The listing builds one solid part. Answer for the finished solid, in the listing's coordinates (mm). Coordinates: 2 decimals unless noted, no trailing zeros. Order: outer loops, then holes, each group sorted by start corner. A loop starts at its lowest first (then second) coordinate and runs counter-clockwise, first axis right, second up.
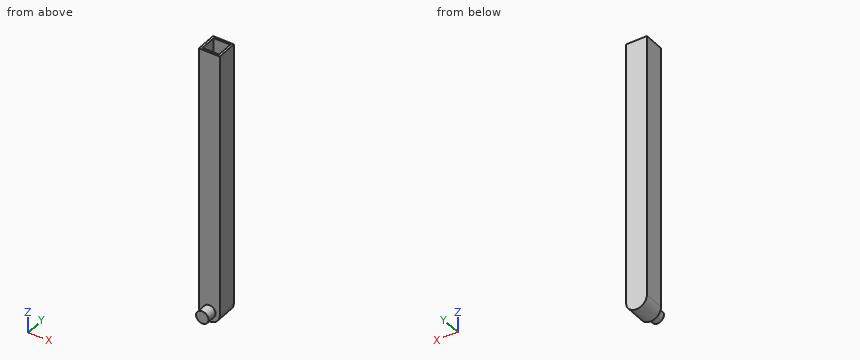
```python
from build123d import *

# Parameters (mm, degrees)
BOSS_EXTRUDE1_DEPTH = 25.4
SKETCH2_W           = 20.32
SKETCH2_H           = 20.32
CUT_EXTRUDE1_DEPTH  = 322.58
SKETCH3_R           = 7.62
BOSS_EXTRUDE2_DEPTH = 12.7


with BuildPart() as part:
    # Sketch1 → Boss-Extrude1 (new body)
    with BuildSketch(Plane(origin=(0, 0, 0), x_dir=(1, 0, 0), z_dir=(0, 1, 0))):
        with BuildLine():
            Line((-12.7, -161.925), (12.7, -161.925))
            Line((12.7, -161.925), (12.7, 161.925))
            ThreePointArc((12.7, 161.925), (0, 174.625), (-12.7, 161.925))
            Line((-12.7, 161.925), (-12.7, -161.925))
        make_face()
    extrude(amount=BOSS_EXTRUDE1_DEPTH)

    # Sketch2 → Cut-Extrude1 (cut)
    with BuildSketch(Plane.XY.offset(161.925)):
        with Locations((0, 12.7)):
            Rectangle(SKETCH2_W, SKETCH2_H)
    extrude(amount=-CUT_EXTRUDE1_DEPTH, mode=Mode.SUBTRACT)

    # Sketch3 → Boss-Extrude2 (add)
    with BuildSketch(Plane.XZ):
        with Locations((0, -161.925)):
            Circle(SKETCH3_R)
    extrude(amount=BOSS_EXTRUDE2_DEPTH)


solid = part.part
```
1) A cutting plane is placed at C-C, the plane y = 8.5. Write down the section's boundary in (x, z) (3 decimals).
2) A cutting plane is placed at D-D, the plane y = -9.5. Write down the section's boundary in (x, z) (3 decimals).
3) Each of these flat-tipped pins is pushed along its axis until it touches: P1, Ø10, axis at x = -2.5, z = -9, coming from the -Y side; P2, Ø4, axis at x = 7, y = -4, coming from the -Z side. Where does it stop, or does it pass through?
4) A cutting plane is placed at B-B, the plane x = 0. Write down the section's boundary in (y, z) (3 decimals).
5) A cutting plane is placed at A-A, the plane z = 134.5. Write down the section's boundary in (x, y).
6) Straight lines are drawn through the part: probe 1 along Y at (x, z) = (-3, 136); probe 2 along X at (y, z) = (20, 95.5); probe 3 along Y at (x, z) = (-11.5, 56.5). For each, find the intervals that lie inside material, in ascending order.
Working result:
1. outline: (-12.7, -161.925) arc R12.7 ccw to (12.7, -161.925) - (12.7, 161.925) - (10.16, 161.925) - (10.16, -160.655) - (-10.16, -160.655) - (-10.16, 161.925) - (-12.7, 161.925) - close
2. outline: circle Ø15.24 at (0, -161.925)
3. P1: stops at y = 0
3. P2: stops at z = -167.68
4. outline: (-12.7, -169.545) - (0, -169.545) - (0, -174.625) - (25.4, -174.625) - (25.4, 161.925) - (22.86, 161.925) - (22.86, -160.655) - (2.54, -160.655) - (2.54, 161.925) - (0, 161.925) - (0, -154.305) - (-12.7, -154.305) - close
5. outline: (-12.7, 0) - (12.7, 0) - (12.7, 25.4) - (-12.7, 25.4) - close; hole (-10.16, 2.54) - (10.16, 2.54) - (10.16, 22.86) - (-10.16, 22.86) - close
6. probe 1: y = 0 to 2.54, 22.86 to 25.4
6. probe 2: x = -12.7 to -10.16, 10.16 to 12.7
6. probe 3: y = 0 to 25.4
